For this review, use the dimensioned drawing (mm, ordinates from the lowest corner) and the shaded views. A direction names the side the tool comes from. Coordinates: 2 decimals unless noted, no trailing zeros. Loops run counter-clockwise (first coordinate to the right, second up) from the corner with the lowest first, then second, coordinate; pieces in that order, holes last. Notation, with made-up numbers: (51, 36) - (81, 36) arc R20 ccw to (81, 64) - close; hole circle Ø10 at (44, 76). An arc over 180 degrees is marked (long way). Return JSON: item names as keys, results as strings. Group by question number.
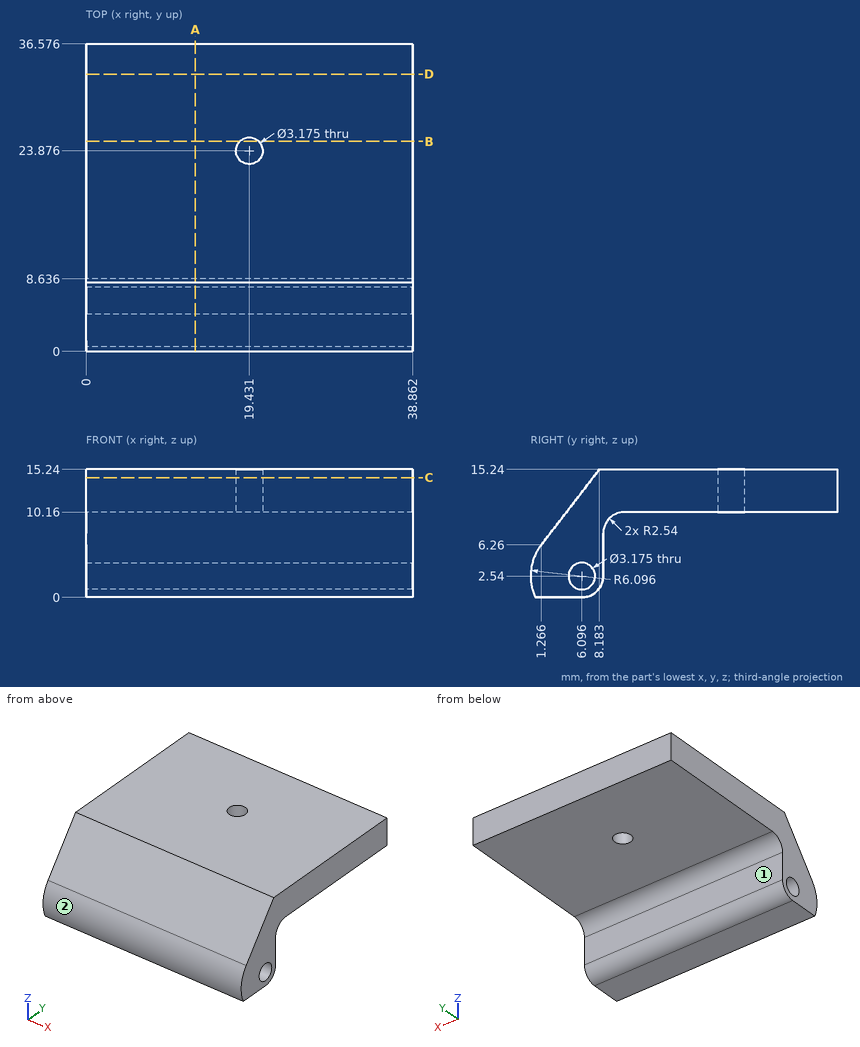
Item 1: Add section D-D (y = 33). State the section outline as (x, z) points.
Item 2: For P1, Ø1.5, axis at x = 9, z = 10.5, coming from the -Y side (1 decimal); P2, Ø1.5, axis at x = 20, y = 10.5, coming from the -Z side; P3, Ø2, axis at x = 29, z = 13, coming from the -Y side; P4, Ø2.5, axis at x = 19.431, y = 23.876, coming from the +Z side (3 decimals), all flat-tipped, find the tip position at first contact; note any pin that passes through.
Item 3: For the marked faces 1 and 2, list the 3-axis set-ups (+Z, -Z, +X, -X, +Y, -Y) from which the entire face can be reached by the end or side of a thin tool; tool diameter is ignored.
Item 4: Add section A-A (x = 13). State the section outline as (y, z) points (1 decimal).
Item 5: To check wall thickness, follow line 1 (Y direction, x = 16, z = 2.5) (1 decimal); line 2 (Z direction, x = 36.5, y = 19); line 3 (Y direction, x = 19, z = 13) (1 decimal). State the ranges of each line that lie inside material, in increasing order. Write a range as from..to.
Item 6: Add section B-B (y = 25). State the section outline as (x, z) points.
Item 7: Add section C-C (z = 14.25). State the section outline as (x, y) points (1 decimal).
Answers below:
{
 "1": {"outline": "(0, 10.16) - (38.86, 10.16) - (38.86, 15.24) - (0, 15.24) - close"},
 "2": {"P1": "stops at y = 4", "P2": "stops at z = 9.72", "P3": "stops at y = 5.69", "P4": "passes through"},
 "3": {"face 1": "-Z, +X, -X, +Y", "face 2": "+X, -X, -Y"},
 "4": {"outline": "(0.6, 0) - (6.1, 0) arc R2.5 ccw to (8.6, 2.5) - (8.6, 7.6) arc R2.5 cw to (11.2, 10.2) - (36.6, 10.2) - (36.6, 15.2) - (8.2, 15.2) - (1.3, 6.3) arc R6.1 ccw to start; hole circle Ø3.2 at (6.1, 2.5)"},
 "5": {"line 1": "y = 0..4.5, 7.7..8.6", "line 2": "z = 10.16..15.24", "line 3": "y = 6.5..22.3, 25.4..36.6"},
 "6": {"outline": "(0, 10.16) - (18.31, 10.16) - (18.31, 15.24) - (0, 15.24) - close; (20.55, 10.16) - (38.86, 10.16) - (38.86, 15.24) - (20.55, 15.24) - close"},
 "7": {"outline": "(0, 7.4) - (38.9, 7.4) - (38.9, 36.6) - (0, 36.6) - close; hole circle Ø3.2 at (19.4, 23.9)"}
}
